Source: three-view drawing plus pictorial views. Frame: mm from the lowest corner of the part. Coordinates: 2 decimals unless noted, no trailing zeros. Write each loop counter-clockwise with the first axis right and the second up, starting at its lowest first coordinate (ties: lowest second). Pieces come first, ordered by that corner, then holes. Notation, with made-up numbers: M 21.25,-35.75 L 31.25,-35.75 A4 ccw 31.25,-31.75 Z; hole C -7.5,-8 d3. An arc over 180 degrees is marked long. Use CSV: the item, a comma, the result in double quotes.
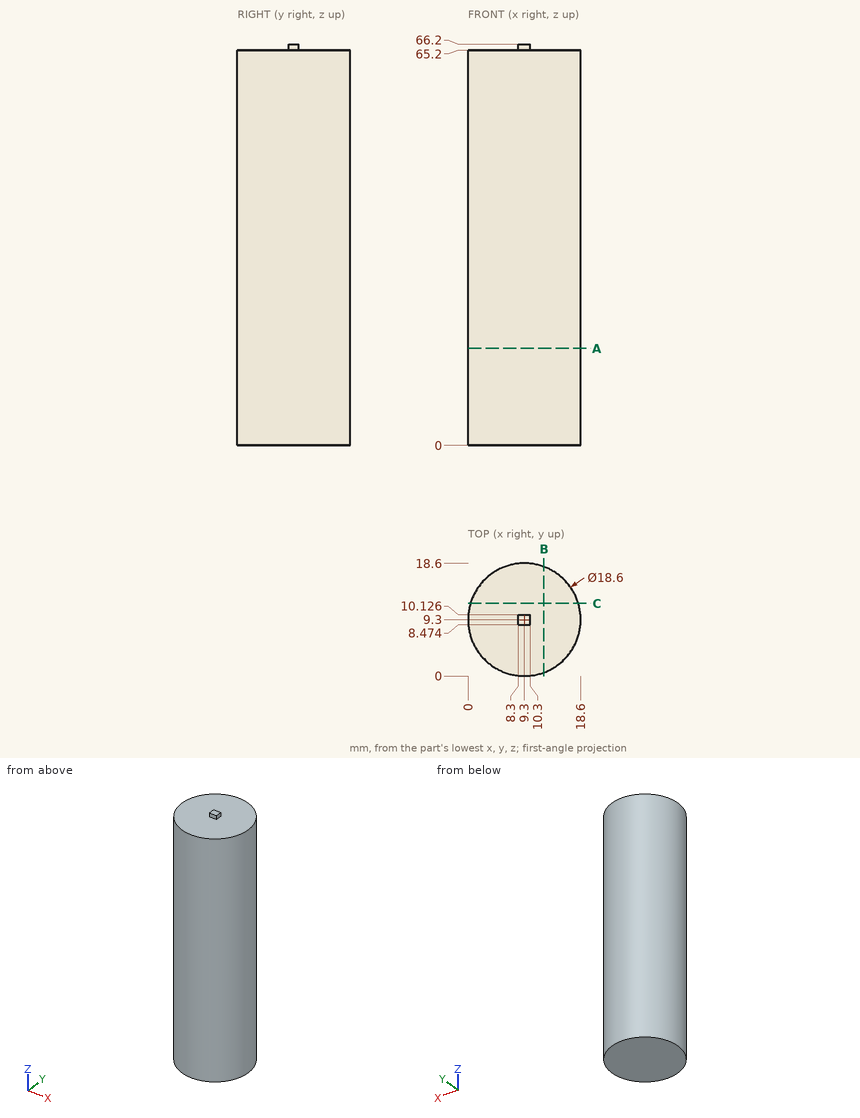
1. Section C-C (y = 12). Return loops of the section in (x, z).
Resolved:
outline,"M 0.4,0 L 18.2,0 L 18.2,65.2 L 0.4,65.2 Z"
2. Material intervals for line 1 (Z direction, x = 7.75, y = 14); line 2 (Y direction, x = 13.5, z = 37), sorted ascending. Write a range as [from, to].
Resolved:
line 1,"z = [0, 65.2]"
line 2,"y = [1, 17.6]"
3. Section A-A (z = 16). Return loops of the section in (x, y), then the cut area to 3 significant figures.
Resolved:
outline,"C 9.3,9.3 d18.6"
area,"272 mm^2"
4. Contact query for flat-ended pins moving along their axis: pin 1 Ø1.1 at (x, z) = (9.5, 65.5) entering from -Y; pin 2 Ø8 at (y, z) = (16.5, 49.5) entering from -X; pin 3 Ø0.5 at (y, z) = (9, 65.5) entering from -X. Output: stop coordinate, or through.
Resolved:
pin 1,"stops at y = 0"
pin 2,"stops at x = 0.57"
pin 3,"stops at x = 8.3"
5. Section B-B (x = 12.5). Return loops of the section in (y, z), then the cut area to 3 significant figures.
Resolved:
outline,"M 0.57,0 L 18.03,0 L 18.03,65.2 L 0.57,65.2 Z"
area,"1,140 mm^2"
